Design review of the part built by this model. Coordinates are the model's own, in mm. Face numbers are marked on the shaded views. A direction names the side the tool comes from. Give positions to 0.01 mm unless a question says otherwise; leave off trailing zeros. Loops run counter-clockwise (first coordinate to the right, second up) from the corner with the lowest first, then second, coordinate; pieces in that order, holes last.
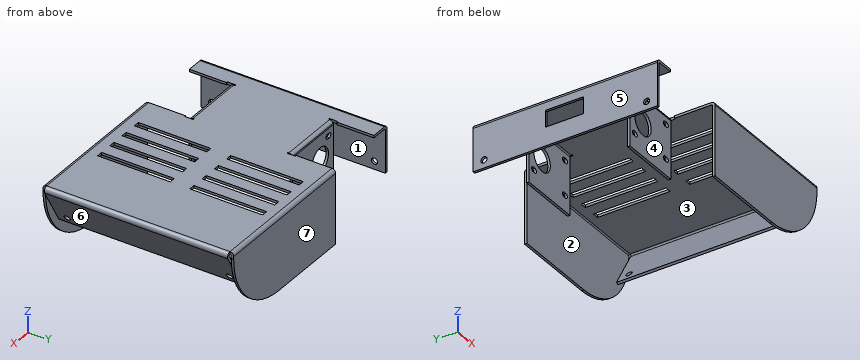
from build123d import *

# Parameters (mm, degrees)
SKETCH7_W                     = 220
SKETCH7_H                     = 150
BASE_FLANGE4_DEPTH            = 2
SKETCH38_W                    = 5
SKETCH38_H                    = 59
CUT_EXTRUDE9_DEPTH            = 10
EDGE_FLANGE9_STRIP_W          = 41
EDGE_FLANGE9_STRIP_H          = 2
EDGE_FLANGE9_STRIP_CUT_DEPTH  = 150
EDGE_FLANGE9_DEPTH            = 150
SKETCH22_W                    = 27.5
SKETCH22_H                    = 30
SKETCH22_W_2                  = 22.5
CUT_EXTRUDE14_DEPTH           = 2
EDGE_FLANGE13_START           = -66
EDGE_FLANGE13_DEPTH           = 52
EDGE_FLANGE13_2_DEPTH         = 1
EDGE_FLANGE13_START_2         = -15
EDGE_FLANGE13_3_DEPTH         = 1
EDGE_FLANGE13_START_3         = -65
EDGE_FLANGE13_4_DEPTH         = 50
EDGE_FLANGE14_START           = -66
EDGE_FLANGE14_DEPTH           = 52
EDGE_FLANGE14_2_DEPTH         = 1
EDGE_FLANGE14_START_2         = -15
EDGE_FLANGE14_3_DEPTH         = 1
EDGE_FLANGE14_START_3         = -65
EDGE_FLANGE14_4_DEPTH         = 50
SKETCH147_W                   = 13.585691309
SKETCH147_H                   = 30.654893209
CUT_EXTRUDE18_DEPTH           = 2
EDGE_FLANGE15_STRIP_W         = 10
EDGE_FLANGE15_STRIP_H         = 2
EDGE_FLANGE15_STRIP_CUT_DEPTH = 125
EDGE_FLANGE15_DEPTH           = 125
EDGE_FLANGE16_DEPTH           = 125
EDGE_FLANGE17_DEPTH           = 149
BREAK_CORNER4_START           = -78
BREAK_CORNER4_DEPTH           = 2
BREAK_CORNER4_START_2         = 75
BREAK_CORNER4_2_DEPTH         = 2
SKETCH164_R                   = 10
CUT_EXTRUDE20_DEPTH           = 176.410946067
SKETCH166_R                   = 2.5
CUT_EXTRUDE21_DEPTH           = 2
SKETCH167_R                   = 2.5
CUT_EXTRUDE24_DEPTH           = 5
SKETCH170_R                   = 2.5
CUT_EXTRUDE25_DEPTH           = 3


# Read off the part's stored shape, not the designer's step: Edge-Flange13, Edge-Flange14, Break-Corner4
# Sheet-metal steps are written as plain solids
with BuildPart() as part:
    # Sketch7 → Base-Flange4 (new body)
    with BuildSketch(Plane.XY):
        Rectangle(SKETCH7_W, SKETCH7_H)
    extrude(amount=-BASE_FLANGE4_DEPTH)

    # Sketch38 → Cut-Extrude9 (cut)
    with BuildSketch(Plane.XY):
        with Locations((12.126416544, -37.5)):
            Rectangle(SKETCH38_W, SKETCH38_H)
        with Locations((27.126416544, -37.5)):
            Rectangle(SKETCH38_W, SKETCH38_H)
        with Locations((42.126416544, -37.5)):
            Rectangle(SKETCH38_W, SKETCH38_H)
        with Locations((57.126416544, -37.5)):
            Rectangle(SKETCH38_W, SKETCH38_H)
        with Locations((57.126416544, 37.5)):
            Rectangle(SKETCH38_W, SKETCH38_H)
        with Locations((42.126416544, 37.5)):
            Rectangle(SKETCH38_W, SKETCH38_H)
        with Locations((27.126416544, 37.5)):
            Rectangle(SKETCH38_W, SKETCH38_H)
        with Locations((12.126416544, 37.5)):
            Rectangle(SKETCH38_W, SKETCH38_H)
    extrude(amount=-CUT_EXTRUDE9_DEPTH, mode=Mode.SUBTRACT)

    # Edge-Flange9 strip (across the edge) → Edge-Flange9 strip cut (cut)
    with BuildSketch(Plane(origin=(-79, -75, -2), x_dir=(1, 0, 0), z_dir=(0, 1, 0))):
        with Locations((-19.5, -1)):
            Rectangle(EDGE_FLANGE9_STRIP_W, EDGE_FLANGE9_STRIP_H)
    extrude(amount=EDGE_FLANGE9_STRIP_CUT_DEPTH, mode=Mode.SUBTRACT)

    # Edge-Flange9 section (across the edge) → Edge-Flange9 (add)
    with BuildSketch(Plane(origin=(-79, -75, -2), x_dir=(1, 0, 0), z_dir=(0, 1, 0))):
        with BuildLine():
            Line((-2, 1), (-2, 36))
            Line((-2, 36), (0, 36))
            Line((0, 36), (0, 1))
            ThreePointArc((0, 1), (0.292893219, 0.292893219), (1, 0))
            Line((1, 0), (1, -2))
            ThreePointArc((1, -2), (-1.121320344, -1.121320344), (-2, 1))
        make_face()
    extrude(amount=EDGE_FLANGE9_DEPTH)

    # Sketch22 → Cut-Extrude14 (cut)
    with BuildSketch(Plane(origin=(0, 0, -2), x_dir=(-1, 0, 0), z_dir=(0, 0, -1))):
        with Locations((51.25, 60)):
            Rectangle(SKETCH22_W, SKETCH22_H)
        with Locations((26.25, 60)):
            Rectangle(SKETCH22_W_2, SKETCH22_H)
        Polygon((65, -45), (37.5, -45), (15, -45), (15, -75), (65, -75), align=None)
    extrude(amount=-CUT_EXTRUDE14_DEPTH, mode=Mode.SUBTRACT)

    # Edge-Flange13 outline → Edge-Flange13 (cut)
    with BuildSketch(Plane.YZ.offset(EDGE_FLANGE13_START)):
        with BuildLine():
            Line((-45, 0), (-45, -2))
            Line((-45, -2), (-41.828427125, -2))
            ThreePointArc((-41.828427125, -2), (-40.732050808, -0.550510257), (-39, 0))
            Line((-39, 0), (-45, 0))
        make_face()
    extrude(amount=EDGE_FLANGE13_DEPTH, mode=Mode.SUBTRACT)

    # Edge-Flange13 2 outline → Edge-Flange13 2 (cut)
    with BuildSketch(Plane.YZ.offset(EDGE_FLANGE13_START)):
        with BuildLine():
            ThreePointArc((-39, 0), (-40.732050808, -0.550510257), (-41.828427125, -2))
            Line((-41.828427125, -2), (-38, -2))
            Line((-38, -2), (-38, 0))
            Line((-38, 0), (-39, 0))
        make_face()
    extrude(amount=EDGE_FLANGE13_2_DEPTH, mode=Mode.SUBTRACT)

    # Edge-Flange13 3 outline → Edge-Flange13 3 (cut)
    with BuildSketch(Plane.YZ.offset(EDGE_FLANGE13_START_2)):
        with BuildLine():
            ThreePointArc((-39, 0), (-40.732050808, -0.550510257), (-41.828427125, -2))
            Line((-41.828427125, -2), (-38, -2))
            Line((-38, -2), (-38, 0))
            Line((-38, 0), (-39, 0))
        make_face()
    extrude(amount=EDGE_FLANGE13_3_DEPTH, mode=Mode.SUBTRACT)

    # Edge-Flange13 4 outline → Edge-Flange13 4 (add)
    with BuildSketch(Plane.YZ.offset(EDGE_FLANGE13_START_3)):
        with BuildLine():
            Line((-39, -2), (-41.828427125, -2))
            ThreePointArc((-41.828427125, -2), (-41.956795679, -2.492694064), (-42, -3))
            Line((-42, -3), (-42, -50))
            Line((-42, -50), (-40, -50))
            Line((-40, -50), (-40, -3))
            ThreePointArc((-40, -3), (-39.707106781, -2.292893219), (-39, -2))
        make_face()
    extrude(amount=EDGE_FLANGE13_4_DEPTH)

    # Edge-Flange14 outline → Edge-Flange14 (cut)
    with BuildSketch(Plane.YZ.offset(EDGE_FLANGE14_START)):
        with BuildLine():
            ThreePointArc((39, 0), (40.732050808, -0.550510257), (41.828427125, -2))
            Line((41.828427125, -2), (45, -2))
            Line((45, -2), (45, 0))
            Line((45, 0), (39, 0))
        make_face()
    extrude(amount=EDGE_FLANGE14_DEPTH, mode=Mode.SUBTRACT)

    # Edge-Flange14 2 outline → Edge-Flange14 2 (cut)
    with BuildSketch(Plane.YZ.offset(EDGE_FLANGE14_START)):
        with BuildLine():
            Line((38, -2), (41.828427125, -2))
            ThreePointArc((41.828427125, -2), (40.732050808, -0.550510257), (39, 0))
            Line((39, 0), (38, 0))
            Line((38, 0), (38, -2))
        make_face()
    extrude(amount=EDGE_FLANGE14_2_DEPTH, mode=Mode.SUBTRACT)

    # Edge-Flange14 3 outline → Edge-Flange14 3 (cut)
    with BuildSketch(Plane.YZ.offset(EDGE_FLANGE14_START_2)):
        with BuildLine():
            Line((38, -2), (41.828427125, -2))
            ThreePointArc((41.828427125, -2), (40.732050808, -0.550510257), (39, 0))
            Line((39, 0), (38, 0))
            Line((38, 0), (38, -2))
        make_face()
    extrude(amount=EDGE_FLANGE14_3_DEPTH, mode=Mode.SUBTRACT)

    # Edge-Flange14 4 outline → Edge-Flange14 4 (add)
    with BuildSketch(Plane.YZ.offset(EDGE_FLANGE14_START_3)):
        with BuildLine():
            Line((40, -3), (40, -50))
            Line((40, -50), (42, -50))
            Line((42, -50), (42, -3))
            ThreePointArc((42, -3), (41.956795679, -2.492694064), (41.828427125, -2))
            Line((41.828427125, -2), (39, -2))
            ThreePointArc((39, -2), (39.707106781, -2.292893219), (40, -3))
        make_face()
    extrude(amount=EDGE_FLANGE14_4_DEPTH)

    # Sketch147 → Cut-Extrude18 (cut)
    with BuildSketch(Plane.ZY.offset(81)):
        with Locations((-16.117047991, 0.696702118)):
            Rectangle(SKETCH147_W, SKETCH147_H)
    extrude(amount=-CUT_EXTRUDE18_DEPTH, mode=Mode.SUBTRACT)

    # Edge-Flange15 strip (across the edge) → Edge-Flange15 strip cut (cut)
    with BuildSketch(Plane(origin=(-15, 75, -2), x_dir=(0, -1, 0), z_dir=(1, 0, 0))):
        with Locations((-4, -1)):
            Rectangle(EDGE_FLANGE15_STRIP_W, EDGE_FLANGE15_STRIP_H)
    extrude(amount=EDGE_FLANGE15_STRIP_CUT_DEPTH, mode=Mode.SUBTRACT)

    # Edge-Flange15 section (across the edge) → Edge-Flange15 (add)
    with BuildSketch(Plane(origin=(-15, 75, -2), x_dir=(0, -1, 0), z_dir=(1, 0, 0))):
        with BuildLine():
            Line((-2, 1), (-2, 58))
            Line((-2, 58), (0, 58))
            Line((0, 58), (0, 1))
            ThreePointArc((0, 1), (0.292893219, 0.292893219), (1, 0))
            Line((1, 0), (1, -2))
            ThreePointArc((1, -2), (-1.121320344, -1.121320344), (-2, 1))
        make_face()
    extrude(amount=EDGE_FLANGE15_DEPTH)

    # Edge-Flange16 section (across the edge) → Edge-Flange16 (add)
    with BuildSketch(Plane(origin=(110, -76, -2), x_dir=(0, 1, 0), z_dir=(-1, 0, 0))):
        with BuildLine():
            Line((-2, 1), (-2, 58))
            Line((-2, 58), (0, 58))
            Line((0, 58), (0, 1))
            ThreePointArc((0, 1), (0.292893219, 0.292893219), (1, 0))
            Line((1, 0), (1, -2))
            ThreePointArc((1, -2), (-1.121320344, -1.121320344), (-2, 1))
        make_face()
    extrude(amount=EDGE_FLANGE16_DEPTH)

    # Edge-Flange17 section (across the edge) → Edge-Flange17 (add)
    with BuildSketch(Plane(origin=(111.732050808, 74, -2), x_dir=(-0.8660254037844398, 0, 0.499999999999998), z_dir=(0, -1, 0))):
        with BuildLine():
            Line((-2, 1.732050808), (-2, 36.535898385))
            Line((-2, 36.535898385), (0, 36.535898385))
            Line((0, 36.535898385), (0, 1.732050808))
            ThreePointArc((0, 1.732050808), (0.5, 0.866025404), (1.5, 0.866025404))
            Line((1.5, 0.866025404), (2.5, -0.866025404))
            ThreePointArc((2.5, -0.866025404), (-0.5, -0.866025404), (-2, 1.732050808))
        make_face()
    extrude(amount=EDGE_FLANGE17_DEPTH)

    # Break-Corner4 outline → Break-Corner4 (cut)
    with BuildSketch(Plane(origin=(0, 0, 0), x_dir=(1, 0, 0), z_dir=(0, 1, 0)).offset(BREAK_CORNER4_START)):
        with BuildLine():
            ThreePointArc((55, 60), (93.890872965, 43.890872965), (110, 5))
            Line((110, 5), (110, 60))
            Line((110, 60), (55, 60))
        make_face()
    extrude(amount=BREAK_CORNER4_DEPTH, mode=Mode.SUBTRACT)

    # Break-Corner4 2 outline → Break-Corner4 2 (cut)
    with BuildSketch(Plane(origin=(0, 0, 0), x_dir=(1, 0, 0), z_dir=(0, 1, 0)).offset(BREAK_CORNER4_START_2)):
        with BuildLine():
            ThreePointArc((55, 60), (93.890872965, 43.890872965), (110, 5))
            Line((110, 5), (110, 60))
            Line((110, 60), (55, 60))
        make_face()
    extrude(amount=BREAK_CORNER4_2_DEPTH, mode=Mode.SUBTRACT)

    # Sketch164 → Cut-Extrude20 (cut, through all)
    with BuildSketch(Plane(origin=(0, 42, 0), x_dir=(1, 0, 0), z_dir=(0, 1, 0))):
        with Locations(Location((-49, 23, 0), (0, 0, 270))):
            Circle(SKETCH164_R)
        with BuildLine():
            Line((-20, 7), (-22, 7))
            ThreePointArc((-22, 7), (-24, 9), (-22, 11))
            Line((-22, 11), (-20, 11))
            ThreePointArc((-20, 11), (-18, 9), (-20, 7))
        make_face()
        with BuildLine():
            Line((-60, 11), (-58, 11))
            ThreePointArc((-58, 11), (-56, 9), (-58, 7))
            Line((-58, 7), (-60, 7))
            ThreePointArc((-60, 7), (-62, 9), (-60, 11))
        make_face()
        with BuildLine():
            Line((-60, 35), (-58, 35))
            ThreePointArc((-58, 35), (-56, 37), (-58, 39))
            Line((-58, 39), (-60, 39))
            ThreePointArc((-60, 39), (-62, 37), (-60, 35))
        make_face()
        with BuildLine():
            Line((-20, 39), (-22, 39))
            ThreePointArc((-22, 39), (-24, 37), (-22, 35))
            Line((-22, 35), (-20, 35))
            ThreePointArc((-20, 35), (-18, 37), (-20, 39))
        make_face()
    extrude(amount=-CUT_EXTRUDE20_DEPTH, mode=Mode.SUBTRACT)

    # Sketch166 → Cut-Extrude21 (cut)
    with BuildSketch(Plane(origin=(86.397114317, 0, -49.881397208), x_dir=(-0.4999999999999983, 0, -0.8660254037844397), z_dir=(0.8660254037844396, 0, -0.4999999999999982))):
        with Locations((-24.152476086, -66)):
            Circle(SKETCH166_R)
    extrude(amount=-CUT_EXTRUDE21_DEPTH, mode=Mode.SUBTRACT)

    # Sketch167 → Cut-Extrude24 (cut)
    with BuildSketch(Plane(origin=(86.397114317, 0, -49.881397208), x_dir=(-0.4999999999999983, 0, -0.8660254037844397), z_dir=(0.8660254037844396, 0, -0.4999999999999982))):
        with Locations((-24.152476086, 66)):
            Circle(SKETCH167_R)
    extrude(amount=-CUT_EXTRUDE24_DEPTH, mode=Mode.SUBTRACT)

    # Sketch170 → Cut-Extrude25 (cut)
    with BuildSketch(Plane.ZY.offset(81)):
        with Locations((-31.38, 66.11)):
            Circle(SKETCH170_R)
        with Locations((-31.38, -66.11)):
            Circle(SKETCH170_R)
    extrude(amount=-CUT_EXTRUDE25_DEPTH, mode=Mode.SUBTRACT)


solid = part.part
Q1. Insertion check: pin 1 (0.6 mm diameter, centred on y = 24, z = -1, fed in from -X); pin 2 (2 mm diameter, centred on x = -38, y = 41, fed in from -Z); pin 3 (3 mm diameter, centred on y = 66.11, z = -31.38, fed in from -X); pin 4 (6 mm diameter, centred on x = -12, y = 5.5, fed in from +Z). Each pin has a flat end and moves straight along its axis. Give the tip position at first contact, or say it passes through.
Results:
pin 1: stops at x = -80.47
pin 2: stops at z = -50
pin 3: stops at x = 93.9
pin 4: stops at z = 0
Q2. Draft analysis for pull direction Y (two halves, no side actions). For the marked faces 5, 6 and 7, state which applies: pulls with the +Y half, pulls with the -Y half, needs draft (parallel to the pull), parting line crosses it, or undercut.
Results:
face 5: needs draft
face 6: undercut
face 7: pulls with the +Y half
Q3. Wall thickness on line 1 (Y direction, x = -80, z = -31); line 2 (Y direction, x = -35, z = -22); line 3 (Y direction, x = 62.5, z = -41.5): over which ranges is each line inside the solid? List them lowest first.
Results:
line 1: y = -75 to -68.58, -63.64 to 63.64, 68.58 to 75
line 2: y = -42 to -40, 40 to 42
line 3: y = -78 to -76, 75 to 77
Q4. Take a section at B-B (y = -22). Give the boundary of the cut face in (x, z).
Results:
outline: (-81, -38) - (-79, -38) - (-79, -3) arc R1 cw to (-78, -2) - (9.63, -2) - (9.63, 0) - (-78, 0) arc R3 ccw to (-81, -3) - close; (14.63, -2) - (24.63, -2) - (24.63, 0) - (14.63, 0) - close; (29.63, -2) - (39.63, -2) - (39.63, 0) - (29.63, 0) - close; (44.63, -2) - (54.63, -2) - (54.63, 0) - (44.63, 0) - close; (59.63, -2) - (110, -2) arc R1 cw to (110.87, -3.5) - (93.46, -33.64) - (95.2, -34.64) - (112.6, -4.5) arc R3 ccw to (110, 0) - (59.63, 0) - close
Q5. Take a section at A-A (x = -49). Give the boundary of the cut face in (y, z).
Results:
outline: (-42, -50) - (-40, -50) - (-40, -33) - (-42, -33) - close; (-42, -13) - (-40, -13) - (-40, -3) arc R1 cw to (-39, -2) - (39, -2) arc R1 cw to (40, -3) - (40, -13) - (42, -13) - (42, -3) arc R3 ccw to (39, 0) - (-39, 0) arc R3 ccw to (-42, -3) - close; (40, -50) - (42, -50) - (42, -33) - (40, -33) - close
Q6. Take a section at C-C (y = -55.5). Give the number of separate pieces and of enclosed holes in the cut face, plus the area to 3 significant figures.
Results:
separate pieces: 6
enclosed holes: 0
area: 390 mm2
Q7. Take a section at D-D (z = -41.5). Give the boundary of the cut face in (x, y).
Results:
outline: (-65, -42) - (-15, -42) - (-15, -40) - (-65, -40) - close; (-65, 40) - (-15, 40) - (-15, 42) - (-65, 42) - close; (-15, -78) - (96.14, -78) - (96.14, -76) - (-15, -76) - close; (-15, 75) - (96.14, 75) - (96.14, 77) - (-15, 77) - close
Q8. Tool access review of the marked faces 1, 2, 3 and 4: name each direction out of +Z, -Z, +X, -X, +Y, -Y from which nothing blocks a thin tool from reaching the whole face with its end or side.
Results:
face 1: -Z, +Y, -Y
face 2: -Z, +X
face 3: none
face 4: +Z, -Z, -Y
